from build123d import *

# Parameters (mm, degrees)
SKIZZE1_W                       = 36.3
SKIZZE1_H                       = 85
AUFSATZ_LINEAR_AUSTRAGEN1_DEPTH = 21.5
WANDUNG1_T                      = -1
SKIZZE4_W                       = 9.03
SKIZZE4_H                       = 3.107106781
SCHNITT_LINEAR_AUSTRAGEN1_DEPTH = 10
SKIZZE8_W                       = 36.3
SKIZZE8_H                       = 85
SKIZZE8_W_2                     = 34.3
SKIZZE8_H_2                     = 83
AUFSATZ_LINEAR_AUSTRAGEN5_DEPTH = 3
VERRUNDUNG1_R                   = 0.9
VERRUNDUNG2_R                   = 1
SKIZZE11_W                      = 34.7
SKIZZE11_H                      = 61.050585676
SCHNITT_LINEAR_AUSTRAGEN5_DEPTH = 20.5
SKIZZE6_W                       = 2.3
SKIZZE6_H                       = 17
SCHNITT_LINEAR_AUSTRAGEN6_DEPTH = 1
AUFSATZ_LINEAR_AUSTRAGEN7_DEPTH = 3
SKIZZE13_R                      = 0.55
SCHNITT_LINEAR_AUSTRAGEN7_DEPTH = 2
SKIZZE14_W                      = 13
SKIZZE14_H                      = 20.1
SCHNITT_LINEAR_AUSTRAGEN8_DEPTH = 3


with BuildPart() as part:
    # Skizze1 → Aufsatz-Linear austragen1 (new body)
    with BuildSketch(Plane.XY):
        with Locations((-18.15, 42.5)):
            Rectangle(SKIZZE1_W, SKIZZE1_H)
    extrude(amount=AUFSATZ_LINEAR_AUSTRAGEN1_DEPTH)

    # Wandung1
    wandung1_openings = [part.faces().sort_by_distance(p)[0] for p in [
        (-18.15, 42.5, 0),
    ]]
    offset(amount=WANDUNG1_T, openings=wandung1_openings, kind=Kind.INTERSECTION)

    # Skizze4 → Schnitt-Linear austragen1 (cut)
    with BuildSketch(Plane(origin=(-35.3, 59.749407146, -1119.925163107), x_dir=(0, -1, 0), z_dir=(1, 0, 0))):
        with Locations((48.249407146, -1137.466609716)):
            Rectangle(SKIZZE4_W, SKIZZE4_H)
    extrude(amount=-SCHNITT_LINEAR_AUSTRAGEN1_DEPTH, mode=Mode.SUBTRACT)

    # Skizze8 → Aufsatz-Linear austragen5 (add)
    with BuildSketch(Plane.XY.offset(21.5)):
        with Locations((-18.15, 42.5)):
            Rectangle(SKIZZE8_W, SKIZZE8_H)
        with Locations((-18.15, 42.5)):
            Rectangle(SKIZZE8_W_2, SKIZZE8_H_2, mode=Mode.SUBTRACT)
    extrude(amount=AUFSATZ_LINEAR_AUSTRAGEN5_DEPTH)

    # Verrundung1
    verrundung1_edges = [part.edges().sort_by_distance(p)[0] for p in [
        (-35.8, 6.985, 15.987893219),
        (-35.8, 6.985, 19.095),
        (-35.8, 16.015, 19.095),
        (-35.8, 16.015, 15.987893219),
    ]]
    fillet(verrundung1_edges, radius=VERRUNDUNG1_R)

    # Verrundung2
    verrundung2_edges = [part.edges().sort_by_distance(p)[0] for p in [
        (-36.3, 85, 12.25),
        (-36.3, 0, 12.25),
        (0, 0, 12.25),
        (0, 85, 12.25),
    ]]
    fillet(verrundung2_edges, radius=VERRUNDUNG2_R)

    # Skizze11 → Schnitt-Linear austragen5 (cut)
    with BuildSketch(Plane(origin=(0, 0, 0), x_dir=(-1, 0, 0), z_dir=(0, 0, -1))):
        with Locations((18.15, 53.474707162)):
            Rectangle(SKIZZE11_W, SKIZZE11_H)
    extrude(amount=-SCHNITT_LINEAR_AUSTRAGEN5_DEPTH, mode=Mode.SUBTRACT)

    # Skizze6 → Schnitt-Linear austragen6 (cut)
    with BuildSketch(Plane(origin=(0, 0, 20.5), x_dir=(-1, 0, 0), z_dir=(0, 0, -1))):
        with Locations((4.15, 11.5)):
            Rectangle(SKIZZE6_W, SKIZZE6_H)
    extrude(amount=-SCHNITT_LINEAR_AUSTRAGEN6_DEPTH, mode=Mode.SUBTRACT)

    # Skizze12 → Aufsatz-Linear austragen7 (add)
    with BuildSketch(Plane.XY.offset(21.5)):
        Polygon((-3, 20), (-5.3, 20), (-5.3, 3), (-33.3, 3), (-33.3, 82), (-3, 82), align=None)
    extrude(amount=AUFSATZ_LINEAR_AUSTRAGEN7_DEPTH)

    # Skizze13 → Schnitt-Linear austragen7 (cut)
    with BuildSketch(Plane(origin=(-2.822587719, 1, -1119.925163107), x_dir=(0, 0, -1), z_dir=(0, 1, 0))):
        with Locations(Location((-1136.220163107, 10.253821552, 0), (0, 0, 180))):
            Circle(SKIZZE13_R)
    extrude(amount=-SCHNITT_LINEAR_AUSTRAGEN7_DEPTH, mode=Mode.SUBTRACT)

    # Skizze14 → Schnitt-Linear austragen8 (cut)
    with BuildSketch(Plane(origin=(-2.822587719, 1, -1119.925163107), x_dir=(0, 0, -1), z_dir=(0, 1, 0))):
        with Locations((-1127.925163107, 15.327412281)):
            Rectangle(SKIZZE14_W, SKIZZE14_H)
    extrude(amount=-SCHNITT_LINEAR_AUSTRAGEN8_DEPTH, mode=Mode.SUBTRACT)


solid = part.part
Geometry: final body of the model. Coordinates: model frame, mm. A direction names the side the tool comes from. Coordinates: 2 decimals unless noted, no trailing zeros. Loops run counter-clockwise (first coordinate to the right, second up) from the corner with the lowest first, then second, coordinate; pieces in that order, holes last. Notation, with made-up numbers: (-22, 48) - (35, 48) arc R20 cw to (35, 82) - close; hole circle Ø3 at (21.5, 83). An arc over 180 degrees is marked (long way). Put each result on its own line as item: value. Start each with the question number.
Q1. Cut plane C-C, the plane y = 64.5. Return loops of the section in (x, z), and give its area (3 significant figures).
Q2. Cut plane D-D, the plane x = -29. Return loops of the section in (y, z).
Q3. Line query: line 1 (Y direction, x = -17.5, z = 21.75); line 2 (Y direction, x = -30, z = 15.25); line 3 (X direction, y = 45.5, z = 11.75). Output: solid intervals per line, ascending.
Q4. Pin query (flat end, axial travel): pin 1 Ø1 at (x, y) = (-10.5, 52) entering from -Z. Return the tip coordinate at first contact, or that it passes through.
Q5. Set-up query: faces 4 (the flat face through (-35.5, 53, 10)), 5 (the flat face through (-1, 42, 23)), 6 (the flat face through (-4, 20, 22)). Return all of +Z, -Z, +X, -X, +Y, -Y with unobstructed straight access to the full face (end or side cutting, diameter ignored); none if empty.
Q6. Cut plane B-B, the plane z = 8.5. Return loops of the section in (x, y), and give its area (3 significant figures).
Q7. Pull-direction query (X, two-part tool) for faces 1 (the flat face through (0, 42, 12)), 2 (the flat face through (-18, 85, 12)), 3 (the flat face through (-3, 51, 23)); classes: released by +X, released by -X, zero draft, split by the parting line, or undercut.
Q8. Cut plane A-A, the plane x = -20. Return loops of the section in (y, z), and give its area (3 significant figures).
Filled sheet:
1. outline: (-36.3, 0) - (-35.5, 0) - (-35.5, 20.5) - (-0.8, 20.5) - (-0.8, 0) - (0, 0) - (0, 24.5) - (-1, 24.5) - (-1, 21.5) - (-3, 21.5) - (-3, 24.5) - (-33.3, 24.5) - (-33.3, 21.5) - (-35.3, 21.5) - (-35.3, 24.5) - (-36.3, 24.5) - close
1. area: 166 mm²
2. outline: (0, 0) - (1, 0) - (1, 20.5) - (84, 20.5) - (84, 0) - (85, 0) - (85, 24.5) - (84, 24.5) - (84, 21.5) - (82, 21.5) - (82, 24.5) - (3, 24.5) - (3, 21.5) - (1, 21.5) - (1, 24.5) - (0, 24.5) - close
3. line 1: 0 to 1, 3 to 82, 84 to 85
3. line 2: 0 to 1, 84 to 85
3. line 3: -36.3 to -35.5, -0.8 to 0
4. pin 1: z = 20.5
5. face 4: -Z
5. face 5: +Z
5. face 6: +Z, -Z
6. outline: (-36.3, 1) arc R1 ccw to (-35.3, 0) - (-28.2, 0) - (-28.2, 1) - (-35.3, 1) - (-35.3, 22.95) - (-35.5, 22.95) - (-35.5, 84) - (-0.8, 84) - (-0.8, 22.95) - (-1, 22.95) - (-1, 1) - (-8.1, 1) - (-8.1, 0) - (-1, 0) arc R1 ccw to (0, 1) - (0, 84) arc R1 ccw to (-1, 85) - (-35.3, 85) arc R1 ccw to (-36.3, 84) - close
6. area: 193 mm²
7. face 1: released by +X
7. face 2: zero draft
7. face 3: undercut
8. outline: (0, 0) - (1, 0) - (1, 1.5) - (0, 1.5) - close; (0, 14.5) - (1, 14.5) - (1, 20.5) - (84, 20.5) - (84, 0) - (85, 0) - (85, 24.5) - (84, 24.5) - (84, 21.5) - (82, 21.5) - (82, 24.5) - (3, 24.5) - (3, 21.5) - (1, 21.5) - (1, 24.5) - (0, 24.5) - close
8. area: 356 mm²
